```python
from build123d import *

# Parameters (mm, degrees)
EXTRUDE_2_DEPTH = 114


with BuildPart() as part:
    # 草图1 → 凸台-拉伸2 (new body)
    with BuildSketch(Plane(origin=(0, 0, 0), x_dir=(1, 0, 0), z_dir=(0, 1, 0))):
        with BuildLine():
            Line((1, 1), (1, 2.775338))
            ThreePointArc((1, 2.775338), (0, 2.95), (-1, 2.775338))
            Line((-1, 2.775338), (-1, 1))
            Line((-1, 1), (-2.775338, 1))
            ThreePointArc((-2.775338, 1), (-2.95, 0), (-2.775338, -1))
            Line((-2.775338, -1), (-1, -1))
            Line((-1, -1), (-1, -2.775338))
            ThreePointArc((-1, -2.775338), (0, -2.95), (1, -2.775338))
            Line((1, -2.775338), (1, -1))
            Line((1, -1), (2.775338, -1))
            ThreePointArc((2.775338, -1), (2.95, 0), (2.775338, 1))
            Line((2.775338, 1), (1, 1))
        make_face()
    extrude(amount=EXTRUDE_2_DEPTH)

    # 草图3 → 旋转3 (revolve)
    with BuildSketch(Plane(origin=(0, 0, 0), x_dir=(0, 0, -1), z_dir=(1, 0, 0))):
        with BuildLine():
            Line((0, 114), (0, 121))
            Line((0, 121), (2.95, 121))
            Line((2.95, 121), (2.95, 120))
            ThreePointArc((2.95, 120), (1.918246, 118.25), (2.95, 116.5))
            Line((2.95, 116.5), (2.95, 114))
            Line((2.95, 114), (0, 114))
        make_face()
        with BuildLine():
            Line((0, 0), (0, -7))
            Line((0, -7), (2.95, -7))
            Line((2.95, -7), (2.95, -6))
            ThreePointArc((2.95, -6), (1.918246, -4.25), (2.95, -2.5))
            Line((2.95, -2.5), (2.95, 0))
            Line((2.95, 0), (0, 0))
        make_face()
    revolve(axis=Axis((0, 0, 0), (0, -1, 0)))


solid = part.part
```
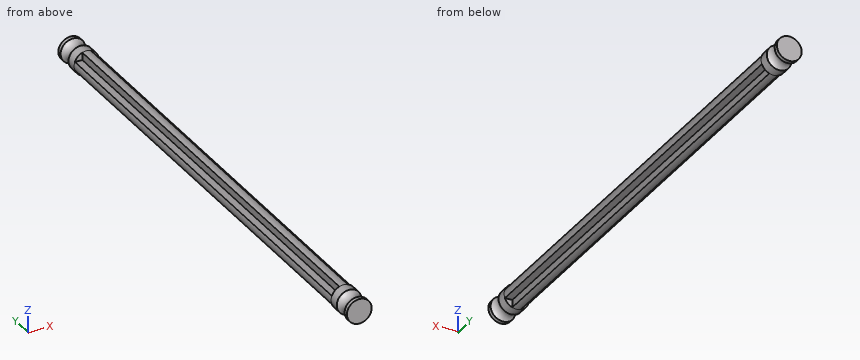
Read the model definition and answer for the solid it produces. Units are mm, in the model's axes. Coordinates: 2 decimals unless noted, no trailing zeros. Write each loop counter-clockwise with the first axis right and the second up, starting at its lowest first coordinate (ties: lowest second). Pieces come first, ordered by that corner, then holes. Notation, with made-up numbers: (77.5, 13) -> (107.5, 13) arc R17 cw to (107.5, 27) -> close; hole circle Ø10 at (58, 14.5). An arc over 180 degrees is marked (long way). Write item = value, one per line.
(1) Straight lines are drawn through the part: L1, parallel to Y at x = -2.45, z = -0.3; L2, parallel to X at y = 94, z = 1.5; L3, parallel to Z at x = 0.2, y = 22. For each, find the intervals that lie inside material, in ascending order. Write a range as from..to.
From the geometry:
L1 = -7..-5.63, -2.87..116.87, 119.63..121
L2 = -1..1
L3 = -2.94..2.94
(2) Section A-A on y = 70.5 is taken. Write down the section's boundary in (x, z), plus the area to 3 significant figures.
From the geometry:
outline = (-2.78, -1) -> (-1, -1) -> (-1, -2.78) arc R2.95 ccw to (1, -2.78) -> (1, -1) -> (2.78, -1) arc R2.95 ccw to (2.78, 1) -> (1, 1) -> (1, 2.78) arc R2.95 ccw to (-1, 2.78) -> (-1, 1) -> (-2.78, 1) arc R2.95 ccw to start
area = 19.1 mm2
(3) Given pin 1 Ø0.5 at (x, y) = (2, 29) entering from +Z; pin 2 Ø1.4 at (x, y) = (2, 73) entering from -Z; pin 3 Ø1.4 at (y, z) = (47.5, 1.5) entering from -X; pin 4 Ø3 at (y, z) = (37.5, -1) entering from +X, each flat-ended and moving along its own axis, determine where each tip first touches the part or whether it passes through.
From the geometry:
pin_1 = 1
pin_2 = -1
pin_3 = -2.84
pin_4 = 2.95
